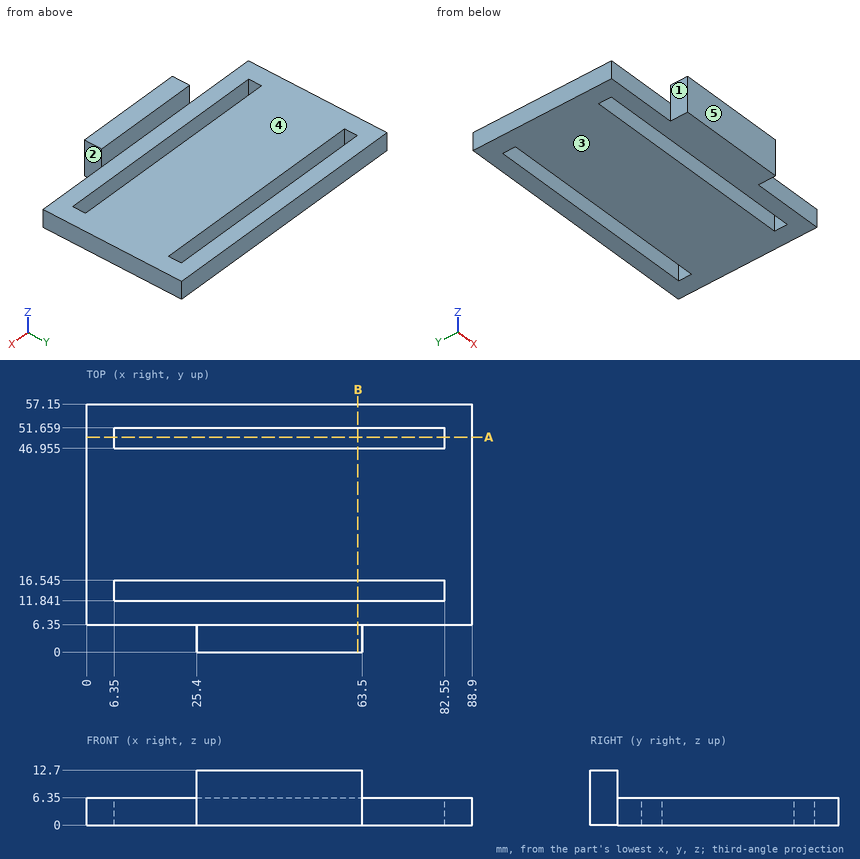
Verification items for this drawing (mm, ordinates from the low corner). A direction names the side the tool comes from. Coordinates: 2 decimals unless noted, no trailing zeros. Write each loop counter-clockwise with the first axis right and the second up, starting at its lowest first coordinate (ties: lowest second). Pieces come first, ordered by that corner, then holes. Notation, with made-up numbers: (87.25, -36) -> (134.25, -36) arc R32 cw to (134.25, -8) -> close; hole circle Ø9 at (47, 60). An arc over 180 degrees is marked (long way). Use CSV: the item, a comma, the result in double quotes. Start each with the question number.
Item 1: Set-up check for the marked faces 1, 2, 3, 4 and 5: record each of +Z, -Z, +X, -X, +Y, -Y from which the full face is reachable in a straight line by a thin tool's end or side.
Item 2: Cross-section at B-B, the plane x = 62.5. State how many separate pieces and enclosed holes the cut face has.
Item 3: Depth check by flat-ended pin: pin 1 Ø12 at (x, y) = (46.5, 34) entering from +Z; pin 2 Ø5 at (y, z) = (3.5, 6.5) entering from -X; pin 3 Ø3 at (x, z) = (76, 4.5) entering from -Y. Enter the tip coordinate at first touch or a pass-through.
Item 4: Thickness scan on line 1 (Z direction, x = 42, y = 44). Record the ranges inside material, lowest first.
Item 5: Cross-section at A-A, the plane y = 49.5. Record the cut outline in (x, z).
Answers:
1,face 1,"+Z, -Z, -X, -Y"
1,face 2,"+Z, -Z, +X, -Y"
1,face 3,"-Z, +X, -X, +Y, -Y"
1,face 4,"+Z, +X, -X, +Y"
1,face 5,"+Z, -Z, +X, -X, -Y"
2,separate pieces,"3"
2,enclosed holes,"0"
3,pin 1,"z = 6.35"
3,pin 2,"x = 25.4"
3,pin 3,"y = 6.35"
4,line 1,"0 to 6.35"
5,outline,"(0, 0) -> (6.35, 0) -> (6.35, 6.35) -> (0, 6.35) -> close; (82.55, 0) -> (88.9, 0) -> (88.9, 6.35) -> (82.55, 6.35) -> close"
